Read the model definition and answer for the solid it produces. Units are mm, in the model's axes. A direction names the side the tool comes from. Round coordinates to 2 decimals unless told otherwise and drop trailing zeros. Write each loop counter-clockwise with the first axis right and the second up, starting at its lowest first coordinate (ties: lowest second). Pieces come first, ordered by that corner, then holes. Notation, with made-up numbers: (-10.5, 79) -> (38.5, 79) arc R16 ccw to (38.5, 109) -> close; hole circle Ø6 at (73, 17). An arc over 180 degrees is marked (long way). Return JSON: item names as keys, results as strings. Group by question number.
(1) A cutting plane is placed at C-C on z = -24. Give the vertices of the cut face in (x, y).
(2) For faces 5 (the flat face through (0, -6.35, 2)), 6 (the flat face through (10.287, -6, -29)), 7 (the cylindrical face through (0.356, -5.837, -19.644)), 8 (the flat face through (0, -3, -20.828)), determine the directions among +Z, -Z, +X, -X, +Y, -Y from which every point of the face is accessible in a straight line to the end or side of a thin tool.
(3) Straight lines are drawn through the part: line 1 (X direction, y = -3, z = -22.5); line 2 (X direction, y = -1.5, z = -29); line 3 (X direction, y = -1.5, z = -27). For each, find the intervals that lie inside material, in ascending order.
(4) Given pin 1 (12 mm diameter, centred on x = -18, y = -21, fed in from +Z); pin 2 (8.5 mm diameter, centred on x = 6, z = -9.5, fed in from -Y); pin 3 (4 mm diameter, centred on x = 6.5, z = 1, fed in from -Y), each flat-ended and moving along its own axis, determine where each tip first touches the part or whether it passes through.
(5) The mould has two halves that part along Z. Classify faces 1 (the flat face through (0, 3.81, -10)), 2 (the flat face through (0, -1, 3.81)), 3 (the cylindrical face through (17.949, -15.027, -29.262)), 4 (the flat face through (0, 0, -9)): released by +Z, released by -Z, zero draft, split by the parting line, or undercut.
(6) A cutting plane is placed at B-B on x = 15.5. Give the vertices of the cut face in (y, z).
(7) A cutting plane is placed at D-D on y = -26.5. Give the vertices of the cut face in (x, z), then the cut area to 3 significant figures.
(8) A cutting plane is placed at A-A on x = -3.5. Give the vertices of the cut face in (y, z).
```python
from build123d import *

# Parameters (mm, degrees)
BOSS_EXTRUDE1_DEPTH = 25.4
BOSS_EXTRUDE2_DEPTH = 10.287
SKETCH4_W           = 12.954
SKETCH4_H           = 7.874
CUT_EXTRUDE1_DEPTH  = 57.596991086
FILLET2_R           = 1.016


with BuildPart() as part:
    # Sketch2 → Boss-Extrude1 (new, symmetric)
    with BuildSketch(Plane(origin=(0, 0, 0), x_dir=(0, 0, -1), z_dir=(1, 0, 0))):
        with BuildLine():
            Line((0, 0), (0, -6.35))
            Line((0, -6.35), (-3.81, -6.35))
            Line((-3.81, -6.35), (-3.81, 3.81))
            Line((-3.81, 3.81), (22.20557735, 3.81))
            ThreePointArc((22.20557735, 3.81), (29.329829331, -15.304797559), (31.75, -35.56))
            Line((31.75, -35.56), (25.4, -35.56))
            ThreePointArc((25.4, -35.56), (23.276174446, -17.292737452), (17.018, 0))
            Line((17.018, 0), (0, 0))
        make_face()
    extrude(amount=BOSS_EXTRUDE1_DEPTH, both=True)

    # Sketch3 → Boss-Extrude2 (add, symmetric)
    with BuildSketch(Plane(origin=(0, 0, 0), x_dir=(0, 0, -1), z_dir=(1, 0, 0))):
        Polygon((31.75, -35.56), (31.75, 3.81), (22.20557735, 3.81), align=None)
    extrude(amount=BOSS_EXTRUDE2_DEPTH, both=True)

    # Sketch4 → Cut-Extrude1 (cut, through all)
    with BuildSketch(Plane(origin=(0, 3.81, 0), x_dir=(1, 0, 0), z_dir=(0, 1, 0))):
        with Locations((0, 24.765)):
            Rectangle(SKETCH4_W, SKETCH4_H)
    extrude(amount=-CUT_EXTRUDE1_DEPTH, mode=Mode.SUBTRACT)

    # Fillet2
    fillet2_edges = [part.edges().sort_by_distance(p)[0] for p in [
        (-6.477, 3.81, -24.765),
        (0, 3.81, -20.828),
        (6.477, 3.81, -24.765),
        (0, 3.81, -28.702),
    ]]
    fillet(fillet2_edges, radius=FILLET2_R)


solid = part.part
```
Checks:
{
 "1": {"outline": "(-25.4, -20.69) -> (-6.48, -20.69) -> (-6.48, 2.79) arc R1.02 ccw to (-7.49, 3.81) -> (-10.29, 3.81) -> (-10.29, 0.11) -> (-25.4, 0.11) -> close; (6.48, -20.69) -> (25.4, -20.69) -> (25.4, 0.11) -> (10.29, 0.11) -> (10.29, 3.81) -> (7.49, 3.81) arc R1.02 ccw to (6.48, 2.79) -> close"},
 "2": {"face 5": "+Z, +X, -X, -Y", "face 6": "-Z, +X, +Y", "face 7": "+X, -X, -Y", "face 8": "+Y, -Y"},
 "3": {"line 1": "x = -25.4 to -6.48, 6.48 to 25.4", "line 2": "x = -10.29 to 10.29", "line 3": "x = -10.29 to -6.48, 6.48 to 10.29"},
 "4": {"pin 1": "stops at z = -22.7", "pin 2": "stops at y = 0", "pin 3": "stops at y = -6.35"},
 "5": {"face 1": "zero draft", "face 2": "released by +Z", "face 3": "released by -Z", "face 4": "undercut"},
 "6": {"outline": "(-35.56, -31.75) arc R85.97 ccw to (3.81, -22.21) -> (3.81, 3.81) -> (-6.35, 3.81) -> (-6.35, 0) -> (0, 0) -> (0, -17.02) arc R79.62 cw to (-35.56, -25.4) -> close"},
 "7": {"outline": "(-25.4, -31.27) -> (-10.29, -31.27) -> (-10.29, -31.75) -> (10.29, -31.75) -> (10.29, -31.27) -> (25.4, -31.27) -> (25.4, -24.88) -> (6.48, -24.88) -> (6.48, -28.7) -> (-6.48, -28.7) -> (-6.48, -24.88) -> (-25.4, -24.88) -> close", "area": "285 mm^2"},
 "8": {"outline": "(-35.56, -31.75) -> (3.81, -31.75) -> (3.81, -29.72) arc R1.02 ccw to (2.79, -28.7) -> (-35.56, -28.7) -> close; (-8.97, -20.83) -> (2.79, -20.83) arc R1.02 ccw to (3.81, -19.81) -> (3.81, 3.81) -> (-6.35, 3.81) -> (-6.35, 0) -> (0, 0) -> (0, -17.02) arc R79.62 cw to start"}
}
